```python
from build123d import *

# Parameters (mm, degrees)
SKETCH1_R          = 1.25
MAIN_DEPTH         = 10
SKETCH2_R          = 1.25
CUT_EXTRUDE1_DEPTH = 21
SKETCH3_R          = 1.25
CUT_EXTRUDE2_DEPTH = 21


with BuildPart() as part:
    # Sketch1 → Main (new body)
    with BuildSketch(Plane.XY):
        Polygon((0, 0), (20, 20), (20, 10), (30, 10), (30, 5), (20, 5), (15, 0), (15, -10), (10, -10), (10, 0), align=None)
        with Locations((15, 5)):
            Circle(SKETCH1_R, mode=Mode.SUBTRACT)
    extrude(amount=MAIN_DEPTH)

    # Sketch2 → Cut-Extrude1 (cut, through all)
    with BuildSketch(Plane(origin=(20, 0, 0), x_dir=(0, 0, -1), z_dir=(1, 0, 0))):
        with Locations((-5, -5)):
            Circle(SKETCH2_R)
        with Locations((-5, 15)):
            Circle(SKETCH2_R)
    extrude(amount=-CUT_EXTRUDE1_DEPTH, mode=Mode.SUBTRACT)

    # Sketch3 → Cut-Extrude2 (cut, through all)
    with BuildSketch(Plane(origin=(0, 0, 0), x_dir=(-1, 0, 0), z_dir=(0, -1, 0))):
        with Locations((-5, -5)):
            Circle(SKETCH3_R)
        with Locations((-25, -5)):
            Circle(SKETCH3_R)
    extrude(amount=-CUT_EXTRUDE2_DEPTH, mode=Mode.SUBTRACT)


solid = part.part
```
Read the model definition and answer for the solid it produces. Units are mm, in the model's axes. A direction names the side the tool comes from. Coordinates: 2 decimals unless noted, no trailing zeros. Order: outer loops, then holes, each group sorted by start corner. A loop starts at its lowest first (then second) coordinate and runs counter-clockwise, first axis right, second up. Notation, with made-up numbers: (-3, 12) - (32, 12) arc R32 ccw to (32, 46) - close; hole circle Ø10 at (-36, 26.5). An arc over 180 degrees is marked (long way). Answer as a JSON object with one key per item and string values. Group by question number.
Item 1: Section B-B (x = 5) is taken. Give the vertices of the cut face in (y, z).
Item 2: Section A-A (z = 5) is taken. Give the vertices of the cut face in (x, y).
Item 3: Section C-C (y = -5) is taken. Give the vertices of the cut face in (x, z).
Item 4: Consider probe 1 along Z at (x, y) = (5, 2.75); probe 2 along Y at (x, z) = (21, 6.75); probe 3 along Y at (x, z) = (18.5, 4.75). Determine where each line is inside the solid, lowest interval first. Write a range as from..to.
Item 5: Flat-ended cylindrical pins translate along their axes: P1, Ø2, axis at y = 6.5, z = 2, coming from the -X side; P2, Ø6, axis at x = 19.5, y = -4, coming from the +Z side; P3, Ø10, axis at x = 4.5, y = -2, coming from the +Z side; P4, Ø5, axis at y = 16.5, z = 3.5, coming from the +X side. Find the tip coordinate at first contact, or state that the pin passes through.
Item 6: Section D-D (z = 1.75) is taken. Give the vertices of the cut face in (x, y).
Item 7: The mould has two halves that part along X. Classify faces 4 (the face through (30, 8, 5)), 5 (the face through (24, 5, 4)), 6 (the face through (6.25, 2.43, 4.95)), 7 (the face through (14.73, 3.78, 4.93)): +X half, -X half, draft (parallel to the pull), parting line (faces both ways), or undercut.
Item 8: A tool of negligible diameter and unlimited length cuts with its end or side. For faces 1 (the face through (6, 0, 4)), 2 (the face through (15, -6, 4)), 3 (the face through (24, 10, 4)), from which of +Z, -Z, +X, -X, +Y, -Y can it reach the whole face along a straight path? Write none if from no direction.
Results are:
{
 "1": {"outline": "(0, 0) - (5, 0) - (5, 3.75) - (0, 3.75) - close; (0, 6.25) - (5, 6.25) - (5, 10) - (0, 10) - close"},
 "2": {"outline": "(0, 0) - (3.75, 0) - (3.75, 3.75) - close; (6.25, 0) - (10, 0) - (10, -3.75) - (15, -3.75) - (15, 0) - (20, 5) - (23.75, 5) - (23.75, 10) - (20, 10) - (20, 13.75) - (13.75, 13.75) - (6.25, 6.25) - close; (10, -10) - (15, -10) - (15, -6.25) - (10, -6.25) - close; (16.25, 16.25) - (20, 16.25) - (20, 20) - close; (26.25, 5) - (30, 5) - (30, 10) - (26.25, 10) - close; hole circle Ø2.5 at (15, 5)"},
 "3": {"outline": "(10, 0) - (15, 0) - (15, 3.75) - (10, 3.75) - close; (10, 6.25) - (15, 6.25) - (15, 10) - (10, 10) - close"},
 "4": {"probe 1": "z = 0..3.75, 6.25..10", "probe 2": "y = 5..10", "probe 3": "y = 3.5..13.78, 16.22..18.5"},
 "5": {"P1": "stops at x = 5.5", "P2": "passes through", "P3": "stops at z = 10", "P4": "stops at x = 20"},
 "6": {"outline": "(0, 0) - (10, 0) - (10, -10) - (15, -10) - (15, 0) - (20, 5) - (30, 5) - (30, 10) - (20, 10) - (20, 20) - close; hole circle Ø2.5 at (15, 5)"},
 "7": {"face 4": "+X half", "face 5": "draft", "face 6": "undercut", "face 7": "undercut"},
 "8": {"face 1": "+Z, -Z, -X, -Y", "face 2": "+Z, -Z, +X, -Y", "face 3": "+Z, -Z, +X, +Y"}
}
